from build123d import *

# Parameters (mm, degrees)
SKETCH_1_W             = 319
SKETCH_1_H             = 122
SM_BASE_FLANGE_1_DEPTH = 1
SKETCH_2_R             = 12.25
CUT_EXTRUDE_1_DEPTH    = 10
SKETCH_3_R             = 1
SKETCH_3_R_2           = 0.707106781
CUT_EXTRUDE_2_DEPTH    = 10
CUT_EXTRUDE_3_DEPTH    = 10
SKETCH_5_R             = 1.25
CUT_EXTRUDE_4_DEPTH    = 10
CHAMFER_1_SIZE         = 1.5
SKETCH_6_W             = 14
SKETCH_6_H             = 13.5
CUT_EXTRUDE_5_DEPTH    = 10


# Sheet-metal steps are written as plain solids
with BuildPart() as part:
    # Sketch 1 → Базовая кромка1 (new body)
    with BuildSketch(Plane.XY):
        with Locations((101.800049421, -35.452668213)):
            Rectangle(SKETCH_1_W, SKETCH_1_H)
    extrude(amount=-SM_BASE_FLANGE_1_DEPTH)

    # Эскиз2 → Вырез-Вытянуть1 (cut)
    with BuildSketch(Plane(origin=(0, 0, -1), x_dir=(-1, 0, 0), z_dir=(0, 0, -1))):
        with Locations((-166.300049421, -35.452668213)):
            Circle(SKETCH_2_R)
        with Locations((-118.300049421, -35.452668213)):
            Circle(SKETCH_2_R)
        with BuildLine():
            ThreePointArc((-222.297668465, -8.271633731), (-221.300049421, -22.702668213), (-220.302430377, -8.271633731))
            ThreePointArc((-220.302430377, -8.271633731), (-221.300049421, -7.202668213), (-222.297668465, -8.271633731))
        make_face()
    extrude(amount=-CUT_EXTRUDE_1_DEPTH, mode=Mode.SUBTRACT)

    # Эскиз3 → Вырез-Вытянуть2 (cut)
    with BuildSketch(Plane(origin=(0, 0, -1), x_dir=(-1, 0, 0), z_dir=(0, 0, -1))):
        with Locations((-179.300049421, -22.452668213)):
            Circle(SKETCH_3_R)
        with Locations((-153.300049421, -22.452668213)):
            Circle(SKETCH_3_R)
        with Locations((-179.300049421, -48.452668213)):
            Circle(SKETCH_3_R)
        with Locations((-153.300049421, -48.452668213)):
            Circle(SKETCH_3_R)
        with Locations((-131.300049421, -48.452668213)):
            Circle(SKETCH_3_R)
        with Locations((-105.300049421, -48.452668213)):
            Circle(SKETCH_3_R_2)
        with Locations((-131.300049421, -22.452668213)):
            Circle(SKETCH_3_R)
        with Locations((-105.300049421, -22.452668213)):
            Circle(SKETCH_3_R)
    extrude(amount=-CUT_EXTRUDE_2_DEPTH, mode=Mode.SUBTRACT)

    # Эскиз4 → Вырез-Вытянуть3 (cut)
    with BuildSketch(Plane(origin=(0, 0, -1), x_dir=(-1, 0, 0), z_dir=(0, 0, -1))):
        Polygon((-213.300049421, -50.101915565), (-207.300049421, -55.452668213), (-207.300049421, -70.452668213), (-235.300049421, -70.452668213), (-235.300049421, -55.452668213), (-229.300049421, -50.101915565), align=None)
    extrude(amount=-CUT_EXTRUDE_3_DEPTH, mode=Mode.SUBTRACT)

    # Эскиз5 → Вырез-Вытянуть4 (cut)
    with BuildSketch(Plane(origin=(0, 0, -1), x_dir=(-1, 0, 0), z_dir=(0, 0, -1))):
        with Locations((-241.300049425, -60.275234132)):
            Circle(SKETCH_5_R)
        with Locations((-201.300049425, -60.275234132)):
            Circle(SKETCH_5_R)
    extrude(amount=-CUT_EXTRUDE_4_DEPTH, mode=Mode.SUBTRACT)

    # Фаска1
    chamfer_1_edges = [part.edges().sort_by_distance(p)[0] for p in [
        (207.300049421, -70.452668213, -0.5),
        (235.300049421, -70.452668213, -0.5),
    ]]
    chamfer(chamfer_1_edges, length=CHAMFER_1_SIZE)

    # Эскиз6 → Вырез-Вытянуть5 (cut)
    with BuildSketch(Plane(origin=(0, 0, -1), x_dir=(-1, 0, 0), z_dir=(0, 0, -1))):
        with Locations((-3.300049421, -66.702668213)):
            Rectangle(SKETCH_6_W, SKETCH_6_H)
    extrude(amount=-CUT_EXTRUDE_5_DEPTH, mode=Mode.SUBTRACT)


solid = part.part
Build history of the part. All positions in model axes, mm. A direction names the side the tool comes from. Round coordinates to 2 decimals unless told otherwise and drop trailing zeros. Write each loop counter-clockwise with the first axis right and the second up, starting at its lowest first coordinate (ties: lowest second). Pieces come first, ordered by that corner, then holes. Notation, with made-up numbers: (24, 18.25) - (74, 18.25) arc R18 ccw to (74, 47.25) - close; hole circle Ø3 at (72.5, 56.5). An arc over 180 degrees is marked (long way). One line per question, with ' | ' between items.
1. Band-saw the part on C-C, the plane x = 124. Write the cut outline in (y, z).
Results are:
outline: (-96.45, -1) - (-46.3, -1) - (-46.3, 0) - (-96.45, 0) - close; (-24.61, -1) - (25.55, -1) - (25.55, 0) - (-24.61, 0) - close
2. Band-saw the part on A-A, the plane y = -65. Write the cut outline in (x, z), and give its area (3 significant figures).
Results are:
outline: (-57.7, -1) - (-3.7, -1) - (-3.7, 0) - (-57.7, 0) - close; (10.3, -1) - (207.3, -1) - (207.3, 0) - (10.3, 0) - close; (235.3, -1) - (261.3, -1) - (261.3, 0) - (235.3, 0) - close | area: 277 mm^2
3. Tool access for faces 1 (the face through (232.342, -52.815, -0.507)), 2 (the face through (100, -35, -1)): list every direction of +Z, -Z, +X, -X, +Y, -Y with a clear straight run to the whole face (end or side of a thin tool).
Results are:
face 1: +Z, -Z | face 2: -Z, +X, -X, +Y, -Y
4. Band-saw the part on B-B, the plane z = -0.7. Give the number of separate pieces and of enclosed holes in the cut face, and give its area (3 significant figures).
Results are:
separate pieces: 1 | enclosed holes: 15 | area: 37,100 mm^2
5. Drop a flat-ended pin along its axis: pin 1 Ø1.6 at (x, y) = (153.3, -48.45) entering from -Z. Give the stop position or say it passes through.
Results are:
pin 1: through
6. Mould opens along Y. For faces 3 (the face through (100, -35, 0)), 4 (the face through (221.605, -22.696, -0.507)) say: released by +Y, released by -Y, zero draft, split by the parting line, or undercut.
Results are:
face 3: zero draft | face 4: undercut
7. Drill centre lines: line 1 along Y through (x, z) = (131, -0.2); line 2 along X through (y, z) = (-68.5, -0.45); line 3 along X through (y, z) = (-49, -0.3). Where is each one in solid material? Low to high. Write a range as from..to.
Results are:
line 1: -96.45..-49.41, -47.5..-23.41, -21.5..25.55 | line 2: -57.7..-3.7, 10.3..207.3, 235.3..261.3 | line 3: -57.7..104.85, 105.75..130.46, 132.14..152.46, 154.14..178.46, 180.14..261.3
